Build history of the part. All positions in model axes, mm. A direction names the side the tool comes from. Give positions to 0.01 mm unless a question says otherwise; leave off trailing zeros. Write each loop counter-clockwise with the first axis right and the second up, starting at its lowest first coordinate (ties: lowest second). Pieces come first, ordered by that corner, then holes. Notation, with made-up numbers: (55, -11.5) -> (83, -11.5) arc R16 ccw to (83, -2.5) -> close; hole circle Ø6 at (28, 74). An arc over 180 degrees is marked (long way). Put each result on its own line as item: value. Start each with the question number.
Item 1: Tool access for faces 1 (the cylindrical face through (-24.21, 14.86, -40.97)), 2 (the cylindrical face through (-25.385, 8.895, 1.014)), 3 (the flat face through (3.096, -19.624, -31.169)), 4 (the flat face through (21.5, 20, -6)), 5 (the flat face through (-21, 20, -49)): list every direction of +Z, -Z, +X, -X, +Y, -Y with a clear straight run to the whole face (end or side of a thin tool).
Item 2: Slice it at B-B, the plane z = -8.5. List the corners of the cut face in (x, y).
Item 3: Drill centre lines: line 1 along Y through (x, z) = (-27, 1); line 2 along Y through (x, z) = (-6, -40); line 3 along Y through (x, z) = (11.5, -14.5). Where is each one in solid material? Low to high.
Item 4: Slice it at A-A, the plane y = 2. List the corners of the cut face in (x, z), plus the area to 3 significant figures.
Item 5: Slice it at C-C, the plane x = -2. List the corners of the cut face in (y, z).
Item 6: Two-plate mould, pull along Y, no slides. Class faces 6 (the flat face through (0, 24, 1)), 7 (the flat face through (-17, -12, -43)), 8 (the flat face through (-9, -21.5, -19)), 9 (the flat face through (-21, -20, -49)): pulls with the +Y half, pulls with the -Y half, needs draft (parallel to the pull), parting line crosses it, or undercut.
Item 7: Flat gauge pins, fed straight in: pin 1 Ø1.1 at (y, z) = (-19, -4) entering from +X; pin 2 Ø4 at (x, y) = (27, 12) entering from +Z; pin 3 Ø15 at (x, z) = (-21, -47.5) entering from -Y; pin 4 Ø14.5 at (x, z) = (3, -14.5) entering from +Y. Where does each tip first touch, or does it go through?
Item 8: Slice it at D-D, the plane x = 27. List the corners of the cut face in (y, z), plus the area to 3 significant figures.
```python
from build123d import *

# Parameters (mm, degrees)
F0_W           = 65
F0_H           = 48
F1_DEPTH       = 2
F2_W           = 49.5
F2_H           = 3.7
F3_DEPTH       = 49
F5_DEPTH       = 58
F6_R           = 25
F7_DEPTH       = 12
F8_R           = 3.5
F9_DEPTH       = 5
F11_R          = 3
F12_DEPTH      = 18
F12_DEPTH_BACK = 18
F13_R          = 25
F14_DEPTH      = 12
F14_DEPTH_BACK = 12


with BuildPart() as f1:
    # F0 (on Top) → F1 (new body)
    with BuildSketch(Plane.XY):
        Rectangle(F0_W, F0_H)
    extrude(amount=F1_DEPTH)

    # F2 (on face) → F3 (join)
    with BuildSketch(Plane(origin=(0, 0, 0), x_dir=(1, 0, 0), z_dir=(0, 0, -1))):
        with Locations((-3.25, 19.65)):
            Rectangle(F2_W, F2_H)
        with Locations((-3.25, -19.65)):
            Rectangle(F2_W, F2_H)
    extrude(amount=F3_DEPTH)

    # F4 (on face) → F5 (cut)
    with BuildSketch(Plane(origin=(0, 21.5, 0), x_dir=(-1, 0, 0), z_dir=(0, 1, 0))):
        Polygon((-21.5, -49), (14.8, -49), (-21.5, -12.831701), align=None)
    extrude(amount=-F5_DEPTH, mode=Mode.SUBTRACT)

    # F8 (on face) → F9 (cut)
    with BuildSketch(Plane.XY.offset(2)):
        with Locations((27, -12)):
            Circle(F8_R)
        with Locations((-27, -12)):
            Circle(F8_R)
        with Locations((-27, 12)):
            Circle(F8_R)
        with Locations((27, 12)):
            Circle(F8_R)
    extrude(amount=-F9_DEPTH, mode=Mode.SUBTRACT)

    # F11 (on Front) → F12 (join, two sides)
    with BuildSketch(Plane.XZ) as f12_sk:
        with Locations((-22, -43)):
            Circle(F11_R)
    extrude(amount=F12_DEPTH)
    extrude(f12_sk.sketch, amount=-F12_DEPTH_BACK)

    # F13 (on Front) → F14 (join, two sides)
    with BuildSketch(Plane.XZ) as f14_sk:
        with Locations((-22, -43)):
            Circle(F13_R)
    extrude(amount=F14_DEPTH)
    extrude(f14_sk.sketch, amount=-F14_DEPTH_BACK)


with BuildPart() as f7:
    # F6 (on Front) → F7 (new body, symmetric)
    with BuildSketch(Plane.XZ):
        with Locations((-22, -43)):
            Circle(F6_R)
    extrude(amount=F7_DEPTH, both=True)


solid = f1.part
```
Values follow:
1. face 1: none
1. face 2: +Z
1. face 3: -Z, +X, -Y
1. face 4: -Z, +X, +Y, -Y
1. face 5: -Z, +X, -X, +Y
2. outline: (-28, -21.5) -> (21.5, -21.5) -> (21.5, -17.8) -> (-28, -17.8) -> close; (-28, 17.8) -> (21.5, 17.8) -> (21.5, 21.5) -> (-28, 21.5) -> close
3. line 1: -24 to -15.5, -8.5 to 8.5, 15.5 to 24
3. line 2: -21.5 to -17.8, -12 to 12, 17.8 to 21.5
3. line 3: -21.5 to -17.8, 17.8 to 21.5
4. outline: circle Ø50 at (-22, -43); (-32.5, 0) -> (32.5, 0) -> (32.5, 2) -> (-32.5, 2) -> close
4. area: 2,090 mm2
5. outline: (-24, 0) -> (-21.5, 0) -> (-21.5, -36.25) -> (-17.8, -36.25) -> (-17.8, 0) -> (17.8, 0) -> (17.8, -36.25) -> (21.5, -36.25) -> (21.5, 0) -> (24, 0) -> (24, 2) -> (-24, 2) -> close; (-12, -58) -> (12, -58) -> (12, -28) -> (-12, -28) -> close
6. face 6: pulls with the +Y half
6. face 7: undercut
6. face 8: pulls with the -Y half
6. face 9: needs draft
7. pin 1: x = 21.5
7. pin 2: through
7. pin 3: y = -21.5
7. pin 4: y = 21.5
8. outline: (-24, 0) -> (-15.5, 0) -> (-15.5, 2) -> (-24, 2) -> close; (-8.5, 0) -> (8.5, 0) -> (8.5, 2) -> (-8.5, 2) -> close; (15.5, 0) -> (24, 0) -> (24, 2) -> (15.5, 2) -> close
8. area: 68.0 mm2
